Autodesk Inventor part; units mm, degrees
ref_plane "YZ Plane" through (0, 0, 0) normal (1, 0, 0) x (0, 1, 0)
ref_plane "XZ Plane" through (0, 0, 0) normal (0, 1, 0) x (-1, 0, 0)
ref_plane "XY Plane" through (0, 0, 0) normal (0, 0, 1) x (1, 0, 0)
sketch "Boceto1" plane through (0, 0, 0) normal (0, 0, 1) x (1, 0, 0)
  line L0 (0, 0) -> (120, 0)
  line L1 (0, 0) -> (0, 40)
  line L2 (0, 40) -> (120, 40)
  line L3 (120, 40) -> (120, 0)
  dimension "d0" = 120
  dimension "d1" = 40
extrude "Extrusión1" add sketch "Boceto1" along normal blind 40
sketch "Boceto2" plane through (0, 0, 40) normal (0, 0, 1) x (1, 0, 0)
  line L0 (0, 0) -> (120, 0) construction
  line L1 (0, 0) -> (30, 0) construction
  line L2 (30, 0) -> (120, 0) construction
  line L3 (120, 0) -> (120, 35.3) construction
  line L4 (120, 0) -> (120, 40) construction
  line L5 (30, 0) -> (120, 0)
  line L6 (120, 35.3) -> (120, 0)
  line L7 (30, 0) -> (30, 5.3)
  line L8 (30, 5.3) -> (120, 35.3)
  line L9 (30, 0) -> (30, 0.3)
  line L10 (30, 0.3) -> (120, 0.3)
  line L11 (30, 0.3) -> (120, 0.3) construction
  dimension "d4" = 30
  dimension "d5" = 35.3
  dimension "d6" = 5.3
  dimension "d46" = 0.3
  dimension "d47" = 90
  dimension "d48" = 0
extrude "Extrusión2" cut sketch "Boceto2" against normal blind 20.3
sketch "Boceto3" plane through (0, 0, 0) normal (0, 0, -1) x (-1, 0, 0)
  line L0 (0, 0) -> (-120, 0) construction
  line L1 (0, 40) -> (0, 0) construction
  line L2 (0, 0) -> (0, 40) construction
  line L3 (0, 0) -> (40, 0) construction
  line L4 (0, 40) -> (-30, 40) construction
  line L5 (-120, 40) -> (0, 40) construction
  line L6 (-30, 40) -> (-30, 34.7)
  line L7 (0, 0) -> (-30, 0) construction
  line L8 (-120, 0) -> (-120, 40)
  line L9 (-30, 0) -> (-120, 0)
  line L10 (-120, 0) -> (-120, 4.7)
  line L11 (-120, 0) -> (-115.3, 0) construction
  line L12 (-120, 4.7) -> (-30, 34.7)
  line L13 (-120, 35.3) -> (-120, 40)
  line L14 (-120, 4.7) -> (-120, 40)
  line L15 (-120, 40) -> (-30, 40)
  dimension "d9" = 40
  dimension "d10" = 90
  dimension "d11" = 30
  dimension "d12" = 5.3
  dimension "d13" = 30
  dimension "d14" = 4.7
  dimension "d15" = 90
extrude "Extrusión3" cut sketch "Boceto3" against normal blind 20.3
sketch "Boceto4" plane through (120, 35.3, 40) normal (1, 0, 0) x (0, 0, -1)
  line L0 (0, 4.7) -> (0, -35.3)
  line L1 (0, 0.386) -> (15.3, 0.386)
  line L2 (0, 0.386) -> (15.3, 0.386) construction
  line L3 (15.3, 0.386) -> (19.7, 0.386)
  line L4 (19.7, 0.386) -> (19.7, 4.486)
  line L5 (19.7, 4.486) -> (15.3, 4.486)
  line L6 (15.3, 4.486) -> (15.3, 0.386)
  line L7 (19.7, 4.7) -> (0, 4.7)
  point P0 (40, -35.3)
  dimension "d18" = 15.3
  dimension "d20" = 4.4
  dimension "d21" = 4.1
  dimension "d49" = 0.214
extrude "Extrusión4" add sketch "Boceto4" along normal blind 5
sketch "Boceto6" plane through (30, 34.7, 0) normal (1, 0, 0) x (0, 0, -1)
  line L0 (0, 0) -> (-20.3, 0)
  line L1 (0, 0) -> (-15, 0)
  line L2 (-15, 0) -> (-20, 0)
  line L3 (-20, 0) -> (-20, 5.3)
  line L4 (-20, 5.3) -> (-15, 5.3)
  line L5 (-15, 5.3) -> (-15, 0)
  point P0 (0, -34.7)
  dimension "d28" = 15
  dimension "d29" = 5
  dimension "d30" = 5.3
extrude "Extrusión6" cut sketch "Boceto6" against normal blind 5
sketch "Boceto7" plane through (30, 0, 40) normal (1, 0, 0) x (0, 0, -1)
  line L0 (20.3, 0) -> (0, 0)
  line L1 (0, 0) -> (15, 0)
  line L2 (15, 0) -> (20, 0)
  line L3 (20, 0) -> (20, 5)
  line L4 (20, 5) -> (15, 5)
  line L5 (15, 5) -> (15, 0)
  point P0 (40, 0)
  dimension "d33" = 15
  dimension "d34" = 5
  dimension "d35" = 5
extrude "Extrusión7" cut sketch "Boceto7" against normal blind 5
sketch "Boceto8" plane through (120, 0, 19.7) normal (1, 0, 0) x (0, 0, -1)
  line L0 (0, 4.7) -> (0, 0)
  line L1 (0, 0) -> (0.3, 0)
  line L2 (0, 0) -> (0.3, 0) construction
  line L3 (0.3, 0) -> (0.3, 0.2)
  line L4 (19.7, 0) -> (-20.3, 0)
  line L5 (0.3, 0) -> (0.5, 0) construction
  line L6 (0.3, 0.2) -> (4.7, 0.2)
  line L7 (4.7, 0.2) -> (4.7, 4.9)
  line L8 (4.7, 4.9) -> (0.3, 4.9)
  line L9 (0.3, 4.9) -> (0.3, 0.2)
  dimension "d38" = 0.3
  dimension "d39" = 0
  dimension "d40" = 0.2
  dimension "d41" = 90
  dimension "d42" = 4.4
  dimension "d43" = 4.7
extrude "Extrusión8" add sketch "Boceto8" along normal blind 5
equation "\"d40\" = Ajuste_02"
equation "\"Ajuste_01\" = 0.1"
equation "\"Ajuste_02\" = 0.2"
equation "\"Ajuste_04\" = 0.4"
equation "\"Ajuste_05\" = 0.5"
properties part number "Hembra_parametrizada"
Source: CAD feature listing. Evaluate the final solid. Frame: model axes, mm. A direction names the side the tool comes from. Give positions to 0.01 mm unless a question says otherwise; leave off trailing zeros. Loops run counter-clockwise (first coordinate to the right, second up) from the corner with the lowest first, then second, coordinate; pieces in that order, holes last. Notation, with made-up numbers: (-13, 44.5) -> (1, 44.5) arc R20 ccw to (1, 49.5) -> close; hole circle Ø9 at (58.25, -36.5). An arc over 180 degrees is marked (long way). Put each result on its own line as item: value. Start each with the question number.
1) Contact query for flat-ended pins moving along their axis: P1, Ø2.5, axis at x = 28.5, z = 23.5, coming from the -Y side; P2, Ø2.5, axis at x = 122.5, y = 2.5, coming from the -Z side; P3, Ø2, axis at x = 123, z = 16.5, coming from the -Y side. Output: stop coordinate, or through.
2) Reachability of faces 4 (the face through (30, 3, 32)), 5 (the face through (28, 2, 20)), 6 (the face through (78, 32, 20.3)), 7 (the face through (122, 38, 24.7)) from +Z, -Z, +X, -X, +Y, -Y: full face, straight path, thin tool, end or side. Return the list, or none.
3) Cut plane D-D (x = 56). Return loops of the section in (y, z), then the cut area to 3 significant figures.
4) Cut plane B-B (x = 104). Return loops of the section in (y, z), then the cut area to 3 significant figures.
5) Draft query along Z for faces 1 (the face through (122, 4.9, 17)), 2 (the face through (28, 3, 25)), 3 (the face through (74, 8, 19.7)). Return one class per face: released by +Z, released by -Z, zero draft, split by the parting line, or undercut.
6) Cut plane A-A (y = 37). Return loops of the section in (x, z).
7) Cut plane C-C (z = 17). Return loops of the section in (x, y).
8) Material intervals for probe 1 along Z at (x, y) = (47, 10); probe 2 along X at (y, z) = (35.5, 5.5); probe 3 along Z at (x, y) = (47, 36.5), sorted ascending.
Results are:
1. P1: stops at y = 5
1. P2: stops at z = 15
1. P3: stops at y = 0.2
2. face 4: +Z, +X, -Y
2. face 5: +X, -Y
2. face 6: -Z, +X, +Y
2. face 7: +Z, +X, +Y, -Y
3. outline: (0, 0) -> (26.03, 0) -> (26.03, 20.3) -> (40, 20.3) -> (40, 40) -> (13.97, 40) -> (13.97, 19.7) -> (0, 19.7) -> close
3. area: 1,030 mm2
4. outline: (0, 0) -> (10.03, 0) -> (10.03, 19.7) -> (0, 19.7) -> close; (29.97, 20.3) -> (40, 20.3) -> (40, 40) -> (29.97, 40) -> close
4. area: 395 mm2
5. face 1: zero draft
5. face 2: undercut
5. face 3: released by +Z
6. outline: (0, 0) -> (30, 0) -> (30, 15) -> (25, 15) -> (25, 20) -> (30, 20) -> (30, 20.3) -> (125, 20.3) -> (125, 24.7) -> (120, 24.7) -> (120, 40) -> (0, 40) -> close
7. outline: (0, 0) -> (120, 0) -> (120, 0.2) -> (125, 0.2) -> (125, 4.9) -> (120, 4.9) -> (120, 4.7) -> (30, 34.7) -> (25, 34.7) -> (25, 40) -> (0, 40) -> close
8. probe 1: z = 0 to 19.7
8. probe 2: x = 0 to 30
8. probe 3: z = 20.3 to 40
